```python
from build123d import *

# Parameters (mm, degrees)
SKETCH2_W                = 25.54
SKETCH2_H                = 25.54
SKETCH2_W_2              = 22.365
SKETCH2_H_2              = 22.365
BOSS_EXTRUDE1_DEPTH      = 50
BOSS_EXTRUDE1_DEPTH_BACK = 50
FILLET1_R                = 1


with BuildPart() as part:
    # Sketch2 → Boss-Extrude1 (new body, two sides)
    with BuildSketch(Plane(origin=(0, 0, 0), x_dir=(0, 0, -1), z_dir=(1, 0, 0))) as boss_extrude1_sk:
        Rectangle(SKETCH2_W, SKETCH2_H)
        Rectangle(SKETCH2_W_2, SKETCH2_H_2, mode=Mode.SUBTRACT)
    extrude(amount=BOSS_EXTRUDE1_DEPTH)
    extrude(boss_extrude1_sk.sketch, amount=-BOSS_EXTRUDE1_DEPTH_BACK)

    # Fillet1
    fillet1_edges = [part.edges().sort_by_distance(p)[0] for p in [
        (0, -12.77, -12.77),
        (0, -12.77, 12.77),
        (0, 12.77, 12.77),
        (0, 12.77, -12.77),
    ]]
    fillet(fillet1_edges, radius=FILLET1_R)


solid = part.part
```
Design review of the part built by this model. Coordinates are the model's own, in mm. A direction names the side the tool comes from. Coordinates: 2 decimals unless noted, no trailing zeros. Write each loop counter-clockwise with the first axis right and the second up, starting at its lowest first coordinate (ties: lowest second). Pieces come first, ordered by that corner, then holes.
1) To check wall thickness, follow L1, parallel to Y at x = -45.5, z = 0.75. State the ranges of the line that lie inside material, in increasing order.
2) Add section A-A (z = 0.5). Write out the cut boundary in (x, y), plus the area to 4 significant figures.
3) Machinability: for faces 1 (the flat face through (1, -11.182, 0)), 2 (the flat face through (-50, 0.1, 11.4)), which of the approach directions +Z, -Z, +X, -X, +Y, -Y give a long, thin tool a straight path to every point of the face, cutting with its end or side? Answer none if there is none.
4) Mouldability with a two-part tool opening along Z and no side actions: class faces 3 (the flat face through (1, 0, -11.182)), 4 (the flat face through (1, 12.77, 0)), 5 (the flat face through (1, 0, 11.182)), 6 (the flat face through (1, 0, -12.77)) as +Z half, -Z half, draft (parallel to the pull), parting line (faces both ways), or undercut.
5) Add section C-C (x = -18). Write out the cut boundary in (y, z), plus the area to 3 significant figures.
Check result:
1. L1: y = -12.77 to -11.18, 11.18 to 12.77
2. outline: (-50, -12.77) - (50, -12.77) - (50, -11.18) - (-50, -11.18) - close; (-50, 11.18) - (50, 11.18) - (50, 12.77) - (-50, 12.77) - close
2. area: 317.5 mm2
3. face 1: +X, -X
3. face 2: +Z, -Z, -X, +Y, -Y
4. face 3: undercut
4. face 4: draft
4. face 5: undercut
4. face 6: -Z half
5. outline: (-12.77, -11.77) arc R1 ccw to (-11.77, -12.77) - (11.77, -12.77) arc R1 ccw to (12.77, -11.77) - (12.77, 11.77) arc R1 ccw to (11.77, 12.77) - (-11.77, 12.77) arc R1 ccw to (-12.77, 11.77) - close; hole (-11.18, -11.18) - (11.18, -11.18) - (11.18, 11.18) - (-11.18, 11.18) - close
5. area: 151 mm2
